```python
from build123d import *

# Parameters (mm, degrees)
BOSS_EXTRUDE1_DEPTH = 46
BOSS_EXTRUDE3_DEPTH = 10
SKETCH17_R          = 1.655
CUT_EXTRUDE10_DEPTH = 30
CUT_EXTRUDE11_DEPTH = 6
CUT_EXTRUDE12_DEPTH = 1.8
CUT_EXTRUDE13_DEPTH = 7.2
SKETCH22_R          = 6.5
BOSS_EXTRUDE4_DEPTH = 10
CUT_EXTRUDE14_DEPTH = 6
CIRPATTERN1_COUNT   = 4
SKETCH24_R          = 6.492418411
CUT_EXTRUDE15_DEPTH = 35


with BuildPart() as part:
    # Sketch1 → Boss-Extrude1 (new body)
    with BuildSketch(Plane.XY):
        with BuildLine():
            Line((-5.05, 9.05), (5.05, 9.05))
            ThreePointArc((5.05, 9.05), (7.878427125, 7.878427125), (9.05, 5.05))
            Line((9.05, 5.05), (9.05, -5.05))
            ThreePointArc((9.05, -5.05), (7.878427125, -7.878427125), (5.05, -9.05))
            Line((5.05, -9.05), (-5.05, -9.05))
            ThreePointArc((-5.05, -9.05), (-7.878427125, -7.878427125), (-9.05, -5.05))
            Line((-9.05, -5.05), (-9.05, 5.05))
            ThreePointArc((-9.05, 5.05), (-7.878427125, 7.878427125), (-5.05, 9.05))
        make_face()
    extrude(amount=BOSS_EXTRUDE1_DEPTH)

    # Sketch15 → Boss-Extrude3 (add)
    with BuildSketch(Plane.XY):
        with BuildLine():
            Line((-5.05, -9.05), (5.05, -9.05))
            ThreePointArc((5.05, -9.05), (7.878427125, -7.878427125), (9.05, -5.05))
            Line((9.05, -5.05), (9.05, 8))
            ThreePointArc((9.05, 8), (7.878427125, 10.828427125), (5.05, 12))
            Line((5.05, 12), (-5.05, 12))
            ThreePointArc((-5.05, 12), (-7.878427125, 10.828427125), (-9.05, 8))
            Line((-9.05, 8), (-9.05, -5.05))
            ThreePointArc((-9.05, -5.05), (-7.878427125, -7.878427125), (-5.05, -9.05))
        make_face()
    extrude(amount=BOSS_EXTRUDE3_DEPTH)

    # Sketch17 → Cut-Extrude10 (cut)
    with BuildSketch(Plane(origin=(9.05, 0, 0), x_dir=(0, 0, -1), z_dir=(1, 0, 0))):
        with Locations((-3.6, 6.1)):
            Circle(SKETCH17_R)
    extrude(amount=-CUT_EXTRUDE10_DEPTH, mode=Mode.SUBTRACT)

    # Sketch18 → Cut-Extrude11 (cut)
    with BuildSketch(Plane.XY):
        Polygon((-4.996539756, -4.259182236), (-3.851088562, -6.946129507), (-2.048481088, -4.559068161), (-0.563070773, -7.21717083), (0.983895836, -4.624244345), (2.704822485, -7.21717083), (3.469678774, -4.870091009), (4.674482161, -7.026054964), (4.998172504, -5.668676456), (4.998172504, 5.373520003), (-4.996539756, 5.373520003), align=None)
    extrude(amount=CUT_EXTRUDE11_DEPTH, mode=Mode.SUBTRACT)

    # Sketch20 → Cut-Extrude12 (cut)
    with BuildSketch(Plane(origin=(0, 0, 6), x_dir=(-1, 0, 0), z_dir=(0, 0, -1))):
        Polygon((-7, 0), (-7, 13.473809321), (7, 13.473809321), (7, 0), (7, -7.194424303), (-7, -7.194424303), align=None)
    extrude(amount=-CUT_EXTRUDE12_DEPTH, mode=Mode.SUBTRACT)

    # Sketch21 → Cut-Extrude13 (cut)
    with BuildSketch(Plane.XY):
        Polygon((5, 17.493725323), (-5, 17.493725323), (-5, 0), (-5, -0.5), (5, -0.5), (5, 0), align=None)
    extrude(amount=CUT_EXTRUDE13_DEPTH, mode=Mode.SUBTRACT)

    # Sketch22 → Boss-Extrude4 (add)
    with BuildSketch(Plane.XY.offset(46)):
        Polygon((-5.006494522, -7.003911735), (4.993505478, -7.003911735), (6.993505478, -5.003911735), (6.993505478, 4.996088265), (4.993505478, 6.996088265), (-5.006494522, 6.996088265), (-7.006494522, 4.996088265), (-7.006494522, -5.003911735), align=None)
        with Locations((-0.006494522, -0.003911735)):
            Circle(SKETCH22_R, mode=Mode.SUBTRACT)
    extrude(amount=BOSS_EXTRUDE4_DEPTH)

    # Sketch23 → Cut-Extrude14 (cut)
    with BuildSketch(Plane.XY.offset(56)):
        Polygon((0, 0), (7, 0.45), (7, -0.45), align=None)
    cut_extrude14 = extrude(amount=-CUT_EXTRUDE14_DEPTH, mode=Mode.SUBTRACT)

    # CirPattern1: Cut-Extrude14 ×4 about axis
    cirpattern1_axis = Axis((-0.006494522, -0.003911735, 0), (0, 0, 1))
    for i in range(1, CIRPATTERN1_COUNT):
        add(cut_extrude14.rotate(cirpattern1_axis, i * 360 / CIRPATTERN1_COUNT), mode=Mode.SUBTRACT)

    # Sketch24 → Cut-Extrude15 (cut)
    with BuildSketch(Plane.XY.offset(46)):
        Circle(SKETCH24_R)
    extrude(amount=-CUT_EXTRUDE15_DEPTH, mode=Mode.SUBTRACT)


solid = part.part
```
Work out the finished part from the listing and answer in its coordinate system (mm). A direction names the side the tool comes from. Round coordinates to 2 decimals unless told otherwise and drop trailing zeros. Loops run counter-clockwise (first coordinate to the right, second up) from the corner with the lowest first, then second, coordinate; pieces in that order, holes last. Notation, with made-up numbers: M 87,-6.75 L 127,-6.75 A34 ccw 127,32.25 Z; hole C 25,23 d8. An arc over 180 degrees is marked long. Use CSV: the item, a comma, the result in double quotes.
Q1. A tool of negligible diameter and unlimited length cuts with its end or side. For faces 1 (the flat face through (-0.1, -7.004, 49.8)), 2 (the flat face through (6.994, -0.1, 49.8)), 3 (the flat face through (6, 3, 6)), 4 (the flat face through (-6, 6, 51)), from which of +Z, -Z, +X, -X, +Y, -Y can it reach the whole face along a straight path? Write none if from no direction.
Determined:
face 1,"+Z, +X, -X, -Y"
face 2,"+Z, +X, +Y, -Y"
face 3,"+Y"
face 4,"+Z, -X, +Y"
Q2. Section A-A, the plane z = 3.6 is taken. State how many separate pieces and enclosed holes the cut face has, then the cut area to 3 significant figures.
Determined:
separate pieces,"3"
enclosed holes,"0"
area,"162 mm2"
Q3. Consider L1, parallel to Z at x = -6, y = -6.5; L2, parallel to Z at x = 6.5, y = 3.75; L3, parallel to Z at x = 4.75, y = -1.5. Determine where each line is inside the solid, lowest interval first.
Determined:
L1,"0 to 6, 7.8 to 46"
L2,"0 to 6, 7.8 to 56"
L3,"7.8 to 11"
Q4. Section B-B, the plane z = 29.5 is taken. Determine the outline of the cut face in (x, y).
Determined:
outline,"M -9.05,-5.05 A4 ccw -5.05,-9.05 L 5.05,-9.05 A4 ccw 9.05,-5.05 L 9.05,5.05 A4 ccw 5.05,9.05 L -5.05,9.05 A4 ccw -9.05,5.05 Z; hole C 0,0 d12.98"
Q5. Each of these flat-tipped pins is pushed along its axis until it touches: pin 1 (1.8 mm diameter, centred on y = 5.5, z = 3.5, fed in from -X); pin 2 (3 mm diameter, centred on y = -1.5, z = 52.5, fed in from +X); pin 3 (5 mm diameter, centred on x = 4.5, z = 49, fed in from +Y). Where does it stop, or does it pass through?
Determined:
pin 1,"through"
pin 2,"x = 6.99"
pin 3,"y = 7"
